Verification items for this drawing (mm, ordinates from the low corner). Round coordinates to 2 decimals unless told otherwise and drop trailing zeros. Loops run counter-clockwise (first coordinate to the right, second up) from the corner with the lowest first, then second, coordinate; pieces in that order, holes last. Notation, with made-up numbers: M 5.5,13 L 38.5,13 A13 ccw 38.5,26 Z; hole C -39,57 d11. An arc over 180 degrees is marked long. Write item = value, one per line. Start each with the question number.
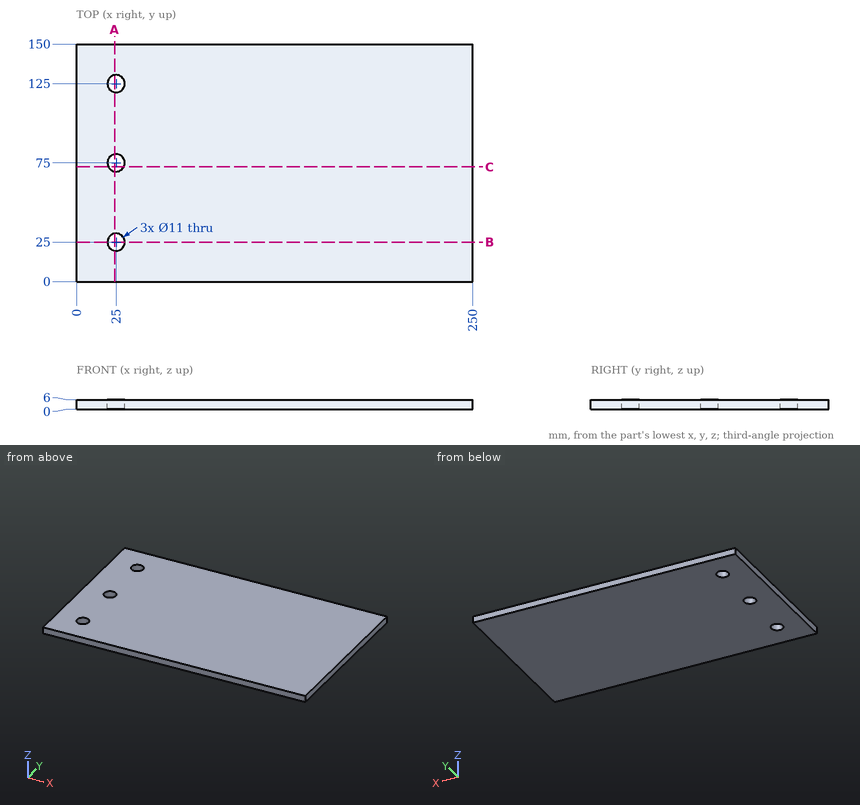
1. Section check B-B, the plane y = 25. Enter the section's corners in (x, z).
2. Section check C-C, the plane y = 72.5. Enter the section's corners in (x, z), and give its area (3 significant figures).
3. Thickness scan on line 1 (Y direction, x = 25, z = 4.45); line 2 (X direction, y = 25, z = 4.85); line 3 (X direction, y = 23, z = 4.55). Record the ranges inside material, lowest first.
4. Section check A-A, the plane x = 24. Enter the section's corners in (y, z).
Computed values:
q1.outline = M 0,0 L 19.5,0 L 19.5,6 L 0,6 Z; M 30.5,0 L 250,0 L 250,6 L 30.5,6 Z
q2.outline = M 0,0 L 20.1,0 L 20.1,6 L 0,6 Z; M 29.9,0 L 250,0 L 250,6 L 29.9,6 Z
q2.area = 1,440 mm2
q3.line_1 = 0 to 19.5, 30.5 to 69.5, 80.5 to 119.5, 130.5 to 150
q3.line_2 = 0 to 19.5, 30.5 to 250
q3.line_3 = 0 to 19.88, 30.12 to 250
q4.outline = M 0,0 L 19.59,0 L 19.59,6 L 0,6 Z; M 30.41,0 L 69.59,0 L 69.59,6 L 30.41,6 Z; M 80.41,0 L 119.59,0 L 119.59,6 L 80.41,6 Z; M 130.41,0 L 150,0 L 150,6 L 130.41,6 Z
